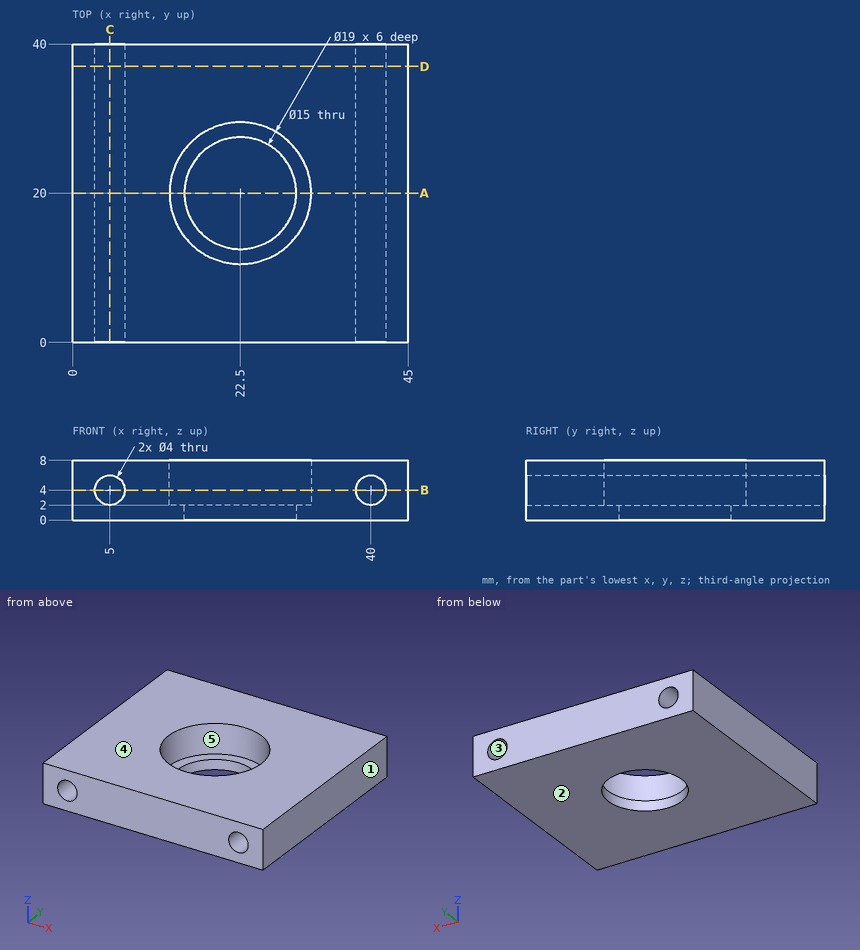
Here's the drawing with two shaded views (mm, measured from the low corner). I have some questions. A direction names the side the tool comes from. Give positions to 0.01 mm unless a question says otherwise; leave off trailing zeros. Order: outer loops, then holes, each group sorted by start corner. A loop starts at its lowest first (then second) coordinate and runs counter-clockwise, first axis right, second up. Notation, with made-up numbers: (-28.75, 57) - (7.25, 57) arc R21 ccw to (7.25, 84) - close; hole circle Ø8 at (53, 26.5). An arc over 180 degrees is marked (long way). Write each question's results on one line, items separated by ' | '.
1) Please list where these lines run through material, in increasing order: line 1 along Y through (x, z) = (22.5, 4.3); line 2 along Z through (x, y) = (5, 2.5); line 3 along Y through (x, z) = (22.5, 0.75). Write a range as [from, to].
Final values:
line 1: y = [0, 10.5], [29.5, 40] | line 2: z = [0, 2], [6, 8] | line 3: y = [0, 12.5], [27.5, 40]
2) On a 3-axis mill with a long thin cutter (end or side, diameter ignored), from which of +Z, -Z, +X, -X, +Y, -Y can I reach the whole of each face in a straight line? I mean the marked faces 4 and 5. Say none if no direction works.
Final values:
face 4: +Z, +X, -X, +Y, -Y | face 5: +Z
3) Suppose I cut it at D-D, the plane y = 37. Write out the boundary of the cut face in (x, z), then the cut area to 3 significant figures.
Final values:
outline: (0, 0) - (45, 0) - (45, 8) - (0, 8) - close; hole circle Ø4 at (5, 4); hole circle Ø4 at (40, 4) | area: 335 mm^2
4) I'm going to push flat-ended pins straight in: pin 1 Ø6 at (x, y) = (11, 16.5) entering from -Z; pin 2 Ø3.5 at (x, z) = (5, 4) entering from -Y. Where does each tip first touch, or does it pass through?
Final values:
pin 1: stops at z = 0 | pin 2: passes through
5) Suppose I cut it at A-A, the plane y = 20. Write out the boundary of the cut face in (x, z).
Final values:
outline: (0, 0) - (15, 0) - (15, 2) - (13, 2) - (13, 8) - (0, 8) - close; (30, 0) - (45, 0) - (45, 8) - (32, 8) - (32, 2) - (30, 2) - close; hole circle Ø4 at (5, 4); hole circle Ø4 at (40, 4)
6) If we mould it in two halves opening along X, with no side actions, what happens to the marked faces 1, 2 and 3? For each: pulls with the +X half, pulls with the -X half, needs draft (parallel to the pull), parting line crosses it, or undercut.
Final values:
face 1: pulls with the +X half | face 2: needs draft | face 3: undercut
7) Suppose I cut it at B-B, the plane z = 4. Write out the boundary of the cut face in (x, y).
Final values:
outline: (0, 0) - (3, 0) - (3, 40) - (0, 40) - close; (7, 0) - (38, 0) - (38, 40) - (7, 40) - close; (42, 0) - (45, 0) - (45, 40) - (42, 40) - close; hole circle Ø19 at (22.5, 20)
8) Suppose I cut it at C-C, the plane x = 5. Write out the boundary of the cut face in (y, z).
Final values:
outline: (0, 0) - (40, 0) - (40, 2) - (0, 2) - close; (0, 6) - (40, 6) - (40, 8) - (0, 8) - close
